```python
from build123d import *

# Parameters (mm, degrees)
BOSS_EXTRUDE1_DEPTH = 5
SKETCH2_W           = 20
SKETCH2_H           = 55
BOSS_EXTRUDE2_DEPTH = 2
FILLET1_R           = 5
CUT_EXTRUDE1_REACH  = 59.446
SKETCH3_R           = 2.65


with BuildPart() as part:
    # Sketch1 → Boss-Extrude1 (new body)
    with BuildSketch(Plane.XY):
        with BuildLine():
            Line((0, 30), (12, 30))
            Line((12, 30), (14, 30))
            Line((14, 30), (14, 23))
            Line((14, 23), (12, 21.8))
            Line((12, 21.8), (10.5, 26))
            Line((10.5, 26), (9, 26))
            Line((9, 26), (9, -10))
            Line((9, -10), (2, -10))
            Line((2, -10), (2, -12))
            Line((2, -12), (2, -13.5))
            Line((2, -13.5), (2, -21))
            Line((2, -21), (3, -21))
            ThreePointArc((3, -21), (4.787066885, -19.89799329), (4.604774071, -17.806391949))
            Line((4.604774071, -17.806391949), (3.691645375, -16.578714862))
            ThreePointArc((3.691645375, -16.578714862), (6.5, -10.989900772), (9.308354625, -16.578714862))
            Line((9.308354625, -16.578714862), (8.395225929, -17.806391949))
            ThreePointArc((8.395225929, -17.806391949), (8.212933115, -19.89799329), (10, -21))
            Line((10, -21), (11, -21))
            Line((11, -21), (11, -19.8))
            Line((11, -19.8), (11, -18.3))
            Line((11, -18.3), (11, -8))
            Line((11, -8), (12.846019189, -5.8))
            Line((12.846019189, -5.8), (14, -7))
            Line((14, -7), (14, -37))
            Line((14, -37), (14, -40))
            Line((14, -40), (14, -43))
            Line((14, -43), (14, -52))
            Line((14, -52), (8, -52))
            Line((8, -52), (8, -49.5))
            Line((8, -49.5), (11, -49.5))
            Line((11, -49.5), (11, -41.5))
            Line((11, -41.5), (11, -40))
            Line((11, -40), (11, -35))
            Line((11, -35), (10, -35))
            ThreePointArc((10, -35), (7.319399673, -33.346989935), (7.592838893, -30.209587923))
            Line((7.592838893, -30.209587923), (8.505967589, -28.981910837))
            ThreePointArc((8.505967589, -28.981910837), (6.5, -24.989900772), (4.494032411, -28.981910837))
            Line((4.494032411, -28.981910837), (5.407161107, -30.209587923))
            ThreePointArc((5.407161107, -30.209587923), (5.680600328, -33.346989935), (3, -35))
            Line((3, -35), (2, -35))
            Line((2, -35), (0, -35))
            Line((0, -35), (0, 30))
        make_face()
        with BuildLine():
            Line((3, -22), (2, -22))
            Line((2, -22), (2, -33.5))
            Line((2, -33.5), (2, -34))
            Line((2, -34), (3, -34))
            ThreePointArc((3, -34), (4.787066885, -32.89799329), (4.604774071, -30.806391949))
            Line((4.604774071, -30.806391949), (3.691645375, -29.578714862))
            ThreePointArc((3.691645375, -29.578714862), (6.5, -23.989900772), (9.308354625, -29.578714862))
            Line((9.308354625, -29.578714862), (8.395225929, -30.806391949))
            ThreePointArc((8.395225929, -30.806391949), (8.212933115, -32.89799329), (10, -34))
            Line((10, -34), (11, -34))
            Line((11, -34), (11, -22))
            Line((11, -22), (10, -22))
            ThreePointArc((10, -22), (7.319399672, -20.346989935), (7.592838893, -17.209587923))
            Line((7.592838893, -17.209587923), (8.505967589, -15.981910837))
            ThreePointArc((8.505967589, -15.981910837), (6.5, -11.989900772), (4.494032411, -15.981910837))
            Line((4.494032411, -15.981910837), (5.407161107, -17.209587923))
            ThreePointArc((5.407161107, -17.209587923), (5.680600328, -20.346989935), (3, -22))
        make_face(mode=Mode.SUBTRACT)
    extrude(amount=BOSS_EXTRUDE1_DEPTH)

    # Sketch2 → Boss-Extrude2 (add)
    with BuildSketch(Plane(origin=(0, 0, 0), x_dir=(0, 0, -1), z_dir=(1, 0, 0))):
        with Locations((-10, 2.5)):
            Rectangle(SKETCH2_W, SKETCH2_H)
    extrude(amount=BOSS_EXTRUDE2_DEPTH)

    # Fillet1
    fillet1_edges = [part.edges().sort_by_distance(p)[0] for p in [
        (1, 30, 20),
        (1, -25, 20),
    ]]
    fillet(fillet1_edges, radius=FILLET1_R)

    # Sketch3 → Cut-Extrude1 (cut, up to next)
    with BuildSketch(Plane(origin=(0, 0, 0), x_dir=(0, 0, -1), z_dir=(1, 0, 0)), mode=Mode.PRIVATE) as cut_extrude1_sk1:
        with Locations(Location((-13, 22, 0), (0, 0, 270))):
            Circle(SKETCH3_R)
    cut_extrude1_tool1 = extrude(cut_extrude1_sk1.sketch, amount=CUT_EXTRUDE1_REACH, mode=Mode.PRIVATE) & part.part
    # Sketch3 → Cut-Extrude1 (cut, up to next)
    with BuildSketch(Plane(origin=(0, 0, 0), x_dir=(0, 0, -1), z_dir=(1, 0, 0)), mode=Mode.PRIVATE) as cut_extrude1_sk2:
        with Locations(Location((-13, -18, 0), (0, 0, 270))):
            Circle(SKETCH3_R)
    cut_extrude1_tool2 = extrude(cut_extrude1_sk2.sketch, amount=CUT_EXTRUDE1_REACH, mode=Mode.PRIVATE) & part.part
    add(cut_extrude1_tool1.solids().sort_by_distance((0, 22, 13))[0], mode=Mode.SUBTRACT)
    add(cut_extrude1_tool2.solids().sort_by_distance((0, -18, 13))[0], mode=Mode.SUBTRACT)


solid = part.part
```
Here's how the part is built. I have some questions about the finished solid (model axes, mm). A direction names the side the tool comes from. Round coordinates to 2 decimals unless told otherwise and drop trailing zeros. Loops run counter-clockwise (first coordinate to the right, second up) from the corner with the lowest first, then second, coordinate; pieces in that order, holes last. Notation, with made-up numbers: (22, 26) -> (67, 26) arc R8 ccw to (67, 40) -> close; hole circle Ø7 at (-13, 8). An arc over 180 degrees is marked (long way). Answer as CSV lines item,"result". Start each with the question number.
1. Imagine slicing it at D-D on y = 14. Write out the boundary of the cut face in (x, z), plus the area to 3 significant figures.
2. For faces 4 (the face through (11, -42, 2)), 5 (the face through (13, 22.4, 2.5)), 6 (the face through (9, 8, 2)), 7 (the face through (11, -52, 2)), which set-ups out of +Z, -Z, +X, -X, +Y, -Y let a thin tool reach every point of the face, with its end or its side?
3. I'm going to push flat-ended pins straight in: P1, Ø4, axis at y = -26.5, z = 17.5, coming from the +X side; P2, Ø1.1, axis at x = 2.5, z = 2, coming from the -Y side; P3, Ø3, axis at x = 1.5, z = 10, coming from the -Y side. Where does each tip first touch, or does it pass through?
4. Imagine slicing it at A-A on y = -9. Write out the boundary of the cut face in (x, z), plus the area to 3 significant figures.
5. I need wall thicknesses on probe 1 along Y at (x, z) = (0.55, 13); probe 2 along Z at (x, y) = (0.7, 22); probe 3 along X at (y, z) = (7.5, 8.75). Which ranges of each line are inside material? Lowest first, please. Write a range as from..to.
6. If we mould it in two halves opening along X, with no side actions, what happens to faces 1 (the face through (7.34, -33.39, 2.46)), 2 (the face through (0.99, 19.55, 14.01)), 3 (the face through (0, -2, 10))? For each: pulls with the +X half, pulls with the -X half, needs draft (parallel to the pull), parting line crosses it, or undercut.
7. Imagine slicing it at C-C on z = 9. Write out the boundary of the cut face in (x, y).
8. Imagine slicing it at B-B on y = -41.5. Write out the boundary of the cut face in (x, z), plus the area to 3 significant figures.
Solution:
1,outline,"(0, 0) -> (9, 0) -> (9, 5) -> (2, 5) -> (2, 20) -> (0, 20) -> close"
1,area,"75.0 mm²"
2,face 4,"+Z, -Z, -X"
2,face 5,"+Z, -Z, +X"
2,face 6,"+Z, -Z"
2,face 7,"+Z, -Z, +X, -X, -Y"
3,P1,"x = 2"
3,P2,"y = -35"
3,P3,"y = -25"
4,outline,"(0, 0) -> (9, 0) -> (9, 5) -> (2, 5) -> (2, 20) -> (0, 20) -> close; (11, 0) -> (14, 0) -> (14, 5) -> (11, 5) -> close"
4,area,"90.0 mm²"
5,probe 1,"-25..-20.65, -15.35..19.35, 24.65..30"
5,probe 2,"0..10.35, 15.65..20"
5,probe 3,"0..2"
6,face 1,"undercut"
6,face 2,"needs draft"
6,face 3,"pulls with the -X half"
7,outline,"(0, -25) -> (2, -25) -> (2, 30) -> (0, 30) -> close"
8,outline,"(11, 0) -> (14, 0) -> (14, 5) -> (11, 5) -> close"
8,area,"15.0 mm²"
